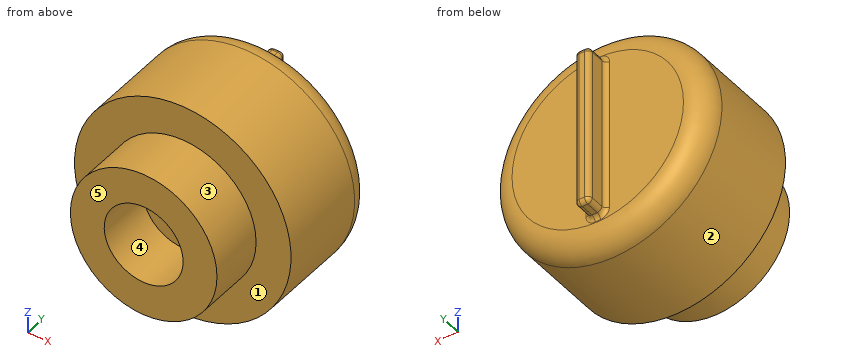
from build123d import *

# Parameters (mm, degrees)
SKETCH1_R           = 3.25
BOSS_EXTRUDE1_DEPTH = 2.46
SKETCH2_R           = 1.75
CUT_EXTRUDE1_DEPTH  = 2.5
SKETCH6_R           = 4.8
BOSS_EXTRUDE2_DEPTH = 5
SKETCH11_W          = 0.64110577
SKETCH11_H          = 7.14375
BOSS_EXTRUDE4_DEPTH = 1
FILLET1_R           = 0.2
FILLET2_R           = 1


with BuildPart() as part:
    # Sketch1 → Boss-Extrude1 (new body)
    with BuildSketch(Plane(origin=(0, 0, 0), x_dir=(1, 0, 0), z_dir=(0, 1, 0))):
        with Locations(Location((0, 0, 0), (0, 0, 270))):
            Circle(SKETCH1_R)
    extrude(amount=BOSS_EXTRUDE1_DEPTH)

    # Sketch2 → Cut-Extrude1 (cut)
    with BuildSketch(Plane.XZ):
        with Locations(Location((0, 0, 0), (0, 0, 270))):
            Circle(SKETCH2_R)
    extrude(amount=-CUT_EXTRUDE1_DEPTH, mode=Mode.SUBTRACT)

    # Sketch6 → Boss-Extrude2 (add)
    with BuildSketch(Plane(origin=(0, 2.46, 0), x_dir=(1, 0, 0), z_dir=(0, 1, 0))):
        with Locations(Location((0, 0, 0), (0, 0, 270))):
            Circle(SKETCH6_R)
    extrude(amount=BOSS_EXTRUDE2_DEPTH)

    # Sketch11 → Boss-Extrude4 (add)
    with BuildSketch(Plane(origin=(0, 7.46, 0), x_dir=(1, 0, 0), z_dir=(0, 1, 0))):
        with Locations((0, -0.015014366)):
            Rectangle(SKETCH11_W, SKETCH11_H)
    extrude(amount=BOSS_EXTRUDE4_DEPTH)

    # Fillet1
    fillet1_edges = [part.edges().sort_by_distance(p)[0] for p in [
        (-0.320552885, 8.46, 0.015014366),
        (-0.320552885, 7.96, -3.556860634),
        (0, 8.46, 3.586889366),
        (-0.320552885, 7.96, 3.586889366),
        (0.320552885, 8.46, 0.015014366),
        (0.320552885, 7.96, 3.586889366),
        (0, 8.46, -3.556860634),
        (0.320552885, 7.96, -3.556860634),
        (-0.320552885, 7.46, 0.015014366),
        (0, 7.46, -3.556860634),
        (0.320552885, 7.46, 0.015014366),
        (0, 7.46, 3.586889366),
    ]]
    fillet(fillet1_edges, radius=FILLET1_R)

    # Fillet2
    fillet2_edges = [part.edges().sort_by_distance(p)[0] for p in [
        (0, 7.46, -4.8),
    ]]
    fillet(fillet2_edges, radius=FILLET2_R)


solid = part.part
The listing builds one solid part. Answer for the finished solid, in the listing's coordinates (mm). Face numbers are marked on the shaded views. A direction names the side the tool comes from. Give positions to 0.01 mm unless a question says otherwise; leave off trailing zeros. Write each loop counter-clockwise with the first axis right and the second up, starting at its lowest first coordinate (ties: lowest second). Pieces come first, ordered by that corner, then holes. Notation, with made-up numbers: (76, 45.25) -> (135, 45.25) arc R25 cw to (135, 73.25) -> close; hole circle Ø9 at (-29.5, 33). An arc over 180 degrees is marked (long way). One line per question, with ' | ' between items. Start each with the question number.
1. For a pull along Z with two mould halves and no side action, classify the marked faces 3, 4 and 5 as pulls with the +Z half, pulls with the -Z half, needs draft (parallel to the pull), parting line crosses it, or undercut.
2. Find the intervals of material crossed by probe 1 along X at (y, z) = (1.7, 0); probe 2 along Y at (x, z) = (-0.75, 1.75); probe 3 along Y at (x, z) = (0.5, 1.25), in increasing order.
3. Section D-D (y = 7) is taken. Determine the outline of the cut face in (x, z).
4. Section A-A (z = 0) is taken. Determine the outline of the cut face in (x, y), plus the area to 3 significant figures.
5. For the marked faces 1 and 2, determine the directions among +Z, -Z, +X, -X, +Y, -Y from which every point of the face is accessible in a straight line to the end or side of a thin tool.
6. Given pin 1 Ø4 at (y, z) = (3.5, -1.5) entering from -X; pin 2 Ø3 at (y, z) = (3.5, 2) entering from +X; pin 3 Ø0.5 at (y, z) = (8, 0.5) entering from +X; pin 4 Ø1.5 at (x, y) = (1.5, 4) entering from +Z, each flat-ended and moving along its own axis, determine where each tip first touches the part or whether it passes through.
7. Section C-C (y = 5) is taken. Determine the outline of the cut face in (x, z), plus the area to 3 significant figures.
8. Section B-B (y = 2.25) is taken. Determine the outline of the cut face in (x, z).
Response values:
1) face 3: parting line crosses it | face 4: undercut | face 5: needs draft
2) probe 1: -3.25 to -1.75, 1.75 to 3.25 | probe 2: 0 to 7.46 | probe 3: 2.46 to 7.46
3) outline: circle Ø9.28 at (0, 0)
4) outline: (-4.8, 2.46) -> (-3.25, 2.46) -> (-3.25, 0) -> (-1.75, 0) -> (-1.75, 2.46) -> (1.75, 2.46) -> (1.75, 0) -> (3.25, 0) -> (3.25, 2.46) -> (4.8, 2.46) -> (4.8, 6.46) arc R1 ccw to (3.8, 7.46) -> (0.52, 7.46) arc R0.2 cw to (0.32, 7.66) -> (0.32, 8.26) arc R0.2 ccw to (0.12, 8.46) -> (-0.12, 8.46) arc R0.2 ccw to (-0.32, 8.26) -> (-0.32, 7.66) arc R0.2 cw to (-0.52, 7.46) -> (-3.8, 7.46) arc R1 ccw to (-4.8, 6.46) -> close | area: 55.6 mm2
5) face 1: -Y | face 2: +Y, -Y
6) pin 1: x = -4.8 | pin 2: x = 4.77 | pin 3: x = 0.32 | pin 4: z = 4.74
7) outline: circle Ø9.6 at (0, 0) | area: 72.4 mm2
8) outline: circle Ø6.5 at (0, 0); hole circle Ø3.5 at (0, 0)
